Part model, mm, in its own coordinate system. Round coordinates to 2 decimals unless told otherwise and drop trailing zeros. Write each loop counter-clockwise with the first axis right and the second up, starting at its lowest first coordinate (ties: lowest second). Pieces come first, ordered by that corner, then holes.
1) Saw through at A-A on x = -238. Write the cut outline in (y, z).
2) Saw through at C-C on z = 11.4. Count the separate pieces of the cut face and the enclosed holes in it, and give its area (3 significant figures).
3) Drill centre lines: L1, parallel to Y at x = -255, z = 11.85; L2, parallel to X at y = 78.5, z = 11.7; L3, parallel to Y at x = -217.5, z = 11.7. Where is each one in solid material? Low to high.
4) Saw through at B-B on y = 173.5. Write the cut outline in (x, z).
5) Flat gauge pins, fed straight in: pin 1 (6.5 mm diameter, centred on x = 215, y = -113.8, fed in from +Z); pin 2 (1.5 mm diameter, centred on y = 211, z = 11.5, fed in from -X); pin 3 (1.5 mm diameter, centred on x = 1.5, z = 13, fed in from +Y); pin 4 (14.5 mm diameter, centred on x = -238, y = 0, fed in from -Z). Where does each tip first touch, or does it go through?
6) Saw through at D-D on x = 95.5. Write the cut outline in (y, z).
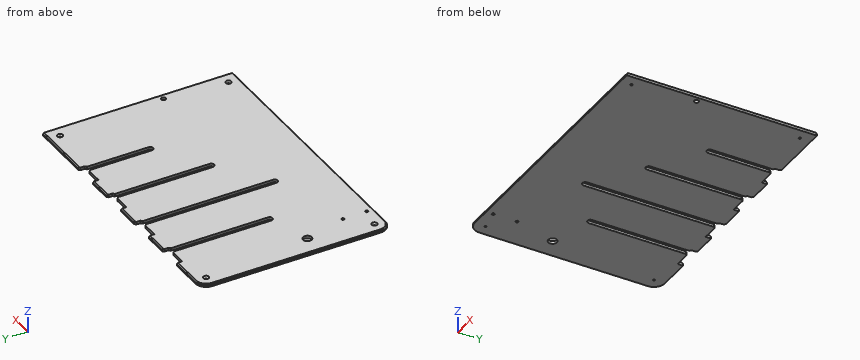
```python
from build123d import *

# Parameters (mm, degrees)
SKETCH018_W     = 510
SKETCH018_H     = 350
PAD015_DEPTH    = 5
SKETCH019_R     = 8
SKETCH019_R_2   = 4.25
POCKET011_DEPTH = 5.001
FILLET005_R     = 20
SKETCH020_R     = 2
POCKET012_DEPTH = 5.001
CHAMFER009_SIZE = 6
CHAMFER010_SIZE = 2
CHAMFER011_SIZE = 3
SKETCH052_W     = 45
SKETCH052_H     = 10
POCKET033_DEPTH = 5.001
CHAMFER024_SIZE = 2.99
SKETCH068_R     = 2.5
POCKET043_DEPTH = 5.001


with BuildPart() as part:
    # Sketch018 → Pad015 (new body)
    with BuildSketch(Plane.XY):
        with Locations((-20, 41.2)):
            Rectangle(SKETCH018_W, SKETCH018_H)
    extrude(amount=PAD015_DEPTH)

    # Sketch019 (on Face6 of Pad015) → Pocket011 (cut, through all)
    with BuildSketch(Plane.XY.offset(5)):
        with Locations((-238, 0)):
            Circle(SKETCH019_R)
        with Locations((225, 0)):
            Circle(SKETCH019_R_2)
        with BuildLine():
            ThreePointArc((-164.573184, 24.404903), (-159.323184, 19.154903), (-154.073184, 24.404903))
            Line((-154.073184, 24.404903), (-154.073184, 216.2))
            ThreePointArc((-154.073184, 216.2), (-159.323184, 221.45), (-164.573184, 216.2))
            Line((-164.573184, 24.404903), (-164.573184, 216.2))
        make_face()
        with BuildLine():
            ThreePointArc((-74.573184, -36.417713), (-69.323184, -41.667713), (-64.073184, -36.417713))
            Line((-64.073184, -36.417713), (-64.073184, 216.2))
            ThreePointArc((-64.073184, 216.2), (-69.323184, 221.45), (-74.573184, 216.2))
            Line((-74.573184, -36.417713), (-74.573184, 216.2))
        make_face()
        with BuildLine():
            ThreePointArc((15.426816, 28.977719), (20.676816, 23.727719), (25.926816, 28.977719))
            Line((25.926816, 28.977719), (25.926816, 216.2))
            ThreePointArc((25.926816, 216.2), (20.676816, 221.45), (15.426816, 216.2))
            Line((15.426816, 28.977719), (15.426816, 216.2))
        make_face()
        with BuildLine():
            ThreePointArc((105.426816, 89.800335), (110.676816, 84.550335), (115.926816, 89.800335))
            Line((115.926816, 89.800335), (115.926816, 216.2))
            ThreePointArc((115.926816, 216.2), (110.676816, 221.45), (105.426816, 216.2))
            Line((105.426816, 89.800335), (105.426816, 216.2))
        make_face()
    extrude(amount=-POCKET011_DEPTH, mode=Mode.SUBTRACT)

    # Fillet005
    fillet005_edges = [part.edges().sort_by_distance(p)[0] for p in [
        (-275, 216.2, 2.5),
        (-275, -133.8, 2.5),
    ]]
    fillet(fillet005_edges, radius=FILLET005_R)

    # Sketch020 (on Face5 of Fillet005) → Pocket012 (cut, through all)
    with BuildSketch(Plane.XY.offset(5)):
        with Locations((-255, 196.2)):
            Circle(SKETCH020_R)
        with Locations((-255, -113.8)):
            Circle(SKETCH020_R)
        with Locations((215, -113.8)):
            Circle(SKETCH020_R)
        with Locations((215, 196.2)):
            Circle(SKETCH020_R)
    extrude(amount=-POCKET012_DEPTH, mode=Mode.SUBTRACT)

    # Chamfer009
    chamfer009_edges = [part.edges().sort_by_distance(p)[0] for p in [
        (-164.573184, 216.2, 2.5),
        (-154.073184, 216.2, 2.5),
        (-74.573184, 216.2, 2.5),
        (-64.073184, 216.2, 2.5),
        (15.426816, 216.2, 2.5),
        (25.926816, 216.2, 2.5),
        (105.426816, 216.2, 2.5),
        (115.926816, 216.2, 2.5),
    ]]
    chamfer(chamfer009_edges, length=CHAMFER009_SIZE)

    # Chamfer010
    chamfer010_edges = [part.edges().sort_by_distance(p)[0] for p in [
        (-212.786592, 216.2, 5),
        (-114.323184, 216.2, 5),
        (-24.323184, 216.2, 5),
        (65.676816, 216.2, 5),
        (178.463408, 216.2, 5),
    ]]
    chamfer(chamfer010_edges, length=CHAMFER010_SIZE)

    # Chamfer011
    chamfer011_edges = [part.edges().sort_by_distance(p)[0] for p in [
        (-257, 196.2, 5),
        (-257, -113.8, 5),
        (213, -113.8, 5),
        (213, 196.2, 5),
    ]]
    chamfer(chamfer011_edges, length=CHAMFER011_SIZE)

    # Sketch052 (on Face1 of Chamfer011) → Pocket033 (cut, through all)
    with BuildSketch(Plane.XY.offset(5)):
        with Locations((-173.573184, 211.2)):
            Rectangle(SKETCH052_W, SKETCH052_H)
        with Locations((-83.573184, 211.2)):
            Rectangle(SKETCH052_W, SKETCH052_H)
        with Locations((6.426816, 211.2)):
            Rectangle(SKETCH052_W, SKETCH052_H)
        with Locations((96.426816, 211.2)):
            Rectangle(SKETCH052_W, SKETCH052_H)
    extrude(amount=-POCKET033_DEPTH, mode=Mode.SUBTRACT)

    # Chamfer024
    chamfer024_edges = [part.edges().sort_by_distance(p)[0] for p in [
        (-164.573184, 206.2, 2.5),
        (-154.073184, 206.2, 2.5),
        (-74.573184, 206.2, 2.5),
        (-64.073184, 206.2, 2.5),
        (15.426816, 206.2, 2.5),
        (25.926816, 206.2, 2.5),
        (105.426816, 206.2, 2.5),
        (115.926816, 206.2, 2.5),
    ]]
    chamfer(chamfer024_edges, length=CHAMFER024_SIZE)

    # Sketch068 (on Face1 of Chamfer024) → Pocket043 (cut, through all)
    with BuildSketch(Plane.XY.offset(5)):
        with Locations((-217.5, -77)):
            Circle(SKETCH068_R)
        with Locations((-217.5, -121)):
            Circle(SKETCH068_R)
    extrude(amount=-POCKET043_DEPTH, mode=Mode.SUBTRACT)


with BuildPart() as part_1:
    # Body011 placement: moved
    add(part.part.moved(Location((0, 0, 10.25))))


solid = part_1.part
```
Completed:
1. outline: (-133.8, 10.25) - (-8, 10.25) - (-8, 15.25) - (-131.8, 15.25) - (-133.8, 13.25) - close; (8, 10.25) - (216.2, 10.25) - (216.2, 13.25) - (214.2, 15.25) - (8, 15.25) - close
2. separate pieces: 1
2. enclosed holes: 8
2. area: 168,000 mm2
3. L1: y = -133.8 to -115.8, -111.8 to 194.2, 198.2 to 216.2
3. L2: x = -275 to -164.57, -154.07 to -74.57, -64.07 to 15.43, 25.93 to 235
3. L3: y = -133.8 to -123.5, -118.5 to -79.5, -74.5 to 216.2
4. outline: (-275, 10.25) - (-164.57, 10.25) - (-164.57, 15.25) - (-273, 15.25) - (-275, 13.25) - close; (-154.07, 10.25) - (-74.57, 10.25) - (-74.57, 15.25) - (-154.07, 15.25) - close; (-64.07, 10.25) - (15.43, 10.25) - (15.43, 15.25) - (-64.07, 15.25) - close; (25.93, 10.25) - (105.43, 10.25) - (105.43, 15.25) - (25.93, 15.25) - close; (115.93, 10.25) - (235, 10.25) - (235, 15.25) - (115.93, 15.25) - close
5. pin 1: stops at z = 13.5
5. pin 2: stops at x = -269.23
5. pin 3: stops at y = 206.2
5. pin 4: passes through
6. outline: (-133.8, 10.25) - (206.2, 10.25) - (206.2, 15.25) - (-131.8, 15.25) - (-133.8, 13.25) - close
